from build123d import *

# Parameters (mm, degrees)
ESQUISSE1_R                  = 67.85
ESQUISSE1_R_2                = 50
BOSS_EXTRU_1_DEPTH           = 71.4
ESQUISSE3_R                  = 135.7
ESQUISSE3_R_2                = 50
BOSS_EXTRU_2_DEPTH           = 64.3
ENL_V_MAT_EXTRU_2_DEPTH      = 236.039294587
ENL_V_MAT_EXTRU_3_DEPTH      = 235.903107685
ENL_V_MAT_EXTRU_3_DEPTH_BACK = 235.903107685
ESQUISSE7_R                  = 7.15
BOSS_EXTRU_3_START           = 53.6
ESQUISSE8_R                  = 182.15
ESQUISSE8_R_2                = 50
BOSS_EXTRU_3_DEPTH           = 53.6


with BuildPart() as part:
    # Esquisse1 → Boss.-Extru.1 (new body)
    with BuildSketch(Plane.XY):
        Circle(ESQUISSE1_R)
        Circle(ESQUISSE1_R_2, mode=Mode.SUBTRACT)
    extrude(amount=-BOSS_EXTRU_1_DEPTH)

    # Esquisse3 → Boss.-Extru.2 (add)
    with BuildSketch(Plane(origin=(0, 0, -71.4), x_dir=(-1, 0, 0), z_dir=(0, 0, -1))):
        Circle(ESQUISSE3_R)
        with Locations(Location((0, 0, 0), (0, 0, 180))):
            Circle(ESQUISSE3_R_2, mode=Mode.SUBTRACT)
    extrude(amount=BOSS_EXTRU_2_DEPTH)

    # Esquisse6 → Enlèv. mat.-Extru.2 (cut, through all)
    with BuildSketch(Plane(origin=(0, 0, -135.7), x_dir=(-1, 0, 0), z_dir=(0, 0, -1))):
        with BuildLine():
            Line((-8, 105.7), (8, 105.7))
            Line((8, 105.7), (8, 135.463980452))
            ThreePointArc((8, 135.463980452), (0, 135.7), (-8, 135.463980452))
            Line((-8, 135.463980452), (-8, 105.7))
        make_face()
        with BuildLine():
            Line((8, -105.7), (8, -135.463980452))
            ThreePointArc((8, -135.463980452), (0, -135.7), (-8, -135.463980452))
            Line((-8, -135.463980452), (-8, -105.7))
            Line((-8, -105.7), (8, -105.7))
        make_face()
    extrude(amount=-ENL_V_MAT_EXTRU_2_DEPTH, mode=Mode.SUBTRACT)

    # Esquisse7 → Enlèv. mat.-Extru.3 (cut, two sides: drawn at the far end of the back side and taken through both)
    with BuildSketch(Plane(origin=(0, 0, 0), x_dir=(0, 0, -1), z_dir=(1, 0, 0)).offset(-ENL_V_MAT_EXTRU_3_DEPTH_BACK)):
        with Locations((103.55, 114.063980452)):
            Circle(ESQUISSE7_R)
        with Locations((103.55, -114.063980452)):
            Circle(ESQUISSE7_R)
    extrude(amount=ENL_V_MAT_EXTRU_3_DEPTH + ENL_V_MAT_EXTRU_3_DEPTH_BACK, mode=Mode.SUBTRACT)

    # Esquisse8 → Boss.-Extru.3 (add)
    with BuildSketch(Plane.XY.offset(BOSS_EXTRU_3_START)):
        Circle(ESQUISSE8_R)
        Circle(ESQUISSE8_R_2, mode=Mode.SUBTRACT)
    extrude(amount=-BOSS_EXTRU_3_DEPTH)


solid = part.part
Build history of the part. All positions in model axes, mm. A direction names the side the tool comes from. Round coordinates to 2 decimals unless told otherwise and drop trailing zeros. Loops run counter-clockwise (first coordinate to the right, second up) from the corner with the lowest first, then second, coordinate; pieces in that order, holes last. Notation, with made-up numbers: (-2, -33.75) -> (29, -33.75) arc R22 cw to (29, -7.75) -> close; hole circle Ø4 at (-29, 75). An arc over 180 degrees is marked (long way). Use CSV: the item, a comma, the result in double quotes. Start each with the question number.
Q1. Flat gauge pins, fed straight in: pin 1 Ø5 at (y, z) = (-72, -53) entering from +X; pin 2 Ø4 at (x, z) = (29, -90.5) entering from +Y; pin 3 Ø9 at (y, z) = (-123.5, -98.5) entering from +X; pin 4 Ø12 at (y, z) = (-18.5, -55.5) entering from -X. Where does each tip first touch, or does it go through?
Q2. Saw through at D-D on z = -60.5. Give the cut face in (x, y), and give its area (3 significant figures).
Q3. Mould opens along Z. For faces 1 (the face through (-8, -124, -104)), 2 (the face through (-28, 62, -71.4)), 3 (the face through (2, -58, -135.7)), 4 (the face through (-37.917, 107.084, -102)) say: +Z half, -Z half, draft (parallel to the pull), parting line (faces both ways), or undercut.
Q4. Drill centre lines: L1, parallel to Z at x = 64, y = -113.5; L2, parallel to Z at x = 109.5, y = 59.5; L3, parallel to Y at x = 0, z = -38.5. Where is each one in solid material? Low to high.
Q5. Saw through at B-B on x = -35.5. Give the cut face in (y, z).
Q6. Saw through at A-A on y = 0. Give the cut face in (x, z).
Q7. Saw through at C-C on z = -103.55. Give the cut face in (x, y).
Q8. Which spindle directions (+Z, -Z, +X, -X, +Y, -Y) get a long thin tool onto all of the face, cutting with end or side? Do faces 5 (the face through (-135.67, -2.87, -103.1)), 6 (the face through (0, 105.7, -104)), 7 (the face through (78, 3, 0)), 8 (the face through (0, -105.7, -104)). Say none if no direction does.
Solutions:
1,pin 1,"passes through"
1,pin 2,"stops at y = 132.99"
1,pin 3,"stops at x = 65.22"
1,pin 4,"stops at x = -66.69"
2,outline,"circle Ø135.7 at (0, 0); hole circle Ø100 at (0, 0)"
2,area,"6,610 mm^2"
3,face 1,"draft"
3,face 2,"undercut"
3,face 3,"-Z half"
3,face 4,"undercut"
4,L1,"z = -135.7 to -110.68, -96.42 to -71.4, 0 to 53.6"
4,L2,"z = -135.7 to -71.4, 0 to 53.6"
4,L3,"y = -67.85 to -50, 50 to 67.85"
5,outline,"(-178.66, 0) -> (-57.82, 0) -> (-57.82, -71.4) -> (-130.97, -71.4) -> (-130.97, -135.7) -> (-35.21, -135.7) -> (-35.21, 53.6) -> (-178.66, 53.6) -> close; (35.21, -135.7) -> (130.97, -135.7) -> (130.97, -71.4) -> (57.82, -71.4) -> (57.82, 0) -> (178.66, 0) -> (178.66, 53.6) -> (35.21, 53.6) -> close; hole circle Ø14.3 at (-114.06, -103.55); hole circle Ø14.3 at (114.06, -103.55)"
6,outline,"(-182.15, 0) -> (-67.85, 0) -> (-67.85, -71.4) -> (-135.7, -71.4) -> (-135.7, -135.7) -> (-50, -135.7) -> (-50, 53.6) -> (-182.15, 53.6) -> close; (50, -135.7) -> (135.7, -135.7) -> (135.7, -71.4) -> (67.85, -71.4) -> (67.85, 0) -> (182.15, 0) -> (182.15, 53.6) -> (50, 53.6) -> close"
7,outline,"(-83.57, -106.91) -> (-8, -106.91) -> (-8, -105.7) -> (8, -105.7) -> (8, -106.91) -> (83.57, -106.91) arc R135.7 ccw to (83.57, 106.91) -> (8, 106.91) -> (8, 105.7) -> (-8, 105.7) -> (-8, 106.91) -> (-83.57, 106.91) arc R135.7 ccw to start; (-61.01, -121.21) arc R135.7 ccw to (-8, -135.46) -> (-8, -121.21) -> close; (-61.01, 121.21) -> (-8, 121.21) -> (-8, 135.46) arc R135.7 ccw to start; (8, -135.46) arc R135.7 ccw to (61.01, -121.21) -> (8, -121.21) -> close; (8, 121.21) -> (61.01, 121.21) arc R135.7 ccw to (8, 135.46) -> close; hole circle Ø100 at (0, 0)"
8,face 5,"-Z, -X"
8,face 6,"-Z, +Y"
8,face 7,"none"
8,face 8,"-Z, -Y"
